Design review of the part built by this model. Coordinates are the model's own, in mm. A direction names the side the tool comes from. Coordinates: 2 decimals unless noted, no trailing zeros. Order: outer loops, then holes, each group sorted by start corner. A loop starts at its lowest first (then second) coordinate and runs counter-clockwise, first axis right, second up.
from build123d import *

# Parameters (mm, degrees)
F0_W     = 19.05
F0_H     = 120.65
F1_DEPTH = 127
F2_W     = 76.2
F2_H     = 76.2
F3_DEPTH = 76.2
F5_D     = 26.19502
F7_D     = 25.4


with BuildPart() as f1:
    # F0 (on Front) → F1 (new body)
    with BuildSketch(Plane.XZ):
        with BuildLine():
            ThreePointArc((120.65, 0), (85.3124331502, 85.3124331502), (0, 120.65))
            Line((0, 120.65), (0, 0))
            Line((0, 0), (120.65, 0))
        make_face()
        with Locations((-9.525, 60.325)):
            Rectangle(F0_W, F0_H)
    extrude(amount=-F1_DEPTH)

    # F2 (on face) → F3 (join)
    with BuildSketch(Plane(origin=(-19.05, 0, 0), x_dir=(0, -1, 0), z_dir=(-1, 0, 0))):
        with Locations((-38.1, 82.55)):
            Rectangle(F2_W, F2_H)
    extrude(amount=F3_DEPTH)

    # F5 (through all)
    with Locations(Plane(origin=(-95.25, 0, 0), x_dir=(0, -1, 0), z_dir=(-1, 0, 0))):
        with Locations((-38.1, 88.9)):
            Hole(F5_D / 2)

    # F7 (through all)
    with Locations(Plane.XZ):
        with Locations((57.15, 44.45)):
            Hole(F7_D / 2)


solid = f1.part
1. Add section D-D (y = 112). Give the boundary of the cut face in (x, z).
2. Add section B-B (x = 57.15). Give the boundary of the cut face in (y, z), and give its area (3 significant figures).
3. For faces 1 (the flat face through (-57, 76.2, 82)), 2 (the flat face through (50, 63, 0)), list the 3-axis set-ups (+Z, -Z, +X, -X, +Y, -Y) from which the entire face can be reached by the end or side of a thin tool; tool diameter is ignored.
4. Add section A-A (y = 38.1). Give the boundary of the cut face in (x, z).
5. Insertion check: pin 1 (4 mm diameter, centred on y = 90.5, z = 32.5, fed in from -X); pin 2 (1 mm diameter, centred on y = 18, z = 63, fed in from +X); pin 3 (5 mm diameter, centred on x = 8.5, z = 75.5, fed in from -Y); pin 4 (10 mm diameter, centred on x = -67.5, y = 25.5, fed in from -Z). Each pin has a flat end and moves straight along its axis. Give the tip position at first contact, or say it passes through.
6. Add section C-C (z = 51). Give the boundary of the cut face in (x, y).
7. To check wall thickness, follow line 1 (Z direction, x = -43.5, y = 38.1); line 2 (Y direction, x = 38, z = 88); line 3 (Z direction, x = 10.5, y = 38.1). State the ranges of each line that lie inside material, in increasing order.
8. Mouldability with a two-part tool opening along Y and no side actions: class faces 3 (the flat face through (-57, 39, 44.45)), 4 (the flat face through (34, 127, 61)), 5 (the cylindrical face through (0.63, 44.14, 77.28)) as pulls with the +Y half, pulls with the -Y half, needs draft (parallel to the pull), parting line crosses it, or undercut.
Solution:
1. outline: (-19.05, 0) - (120.65, 0) arc R120.65 ccw to (0, 120.65) - (-19.05, 120.65) - close; hole circle Ø25.4 at (57.15, 44.45)
2. outline: (0, 0) - (127, 0) - (127, 31.75) - (0, 31.75) - close; (0, 57.15) - (127, 57.15) - (127, 106.26) - (0, 106.26) - close; hole circle Ø26.2 at (38.1, 88.9)
2. area: 9,730 mm2
3. face 1: +Z, -Z, -X, +Y
3. face 2: -Z, +X, -X, +Y, -Y
4. outline: (-95.25, 44.45) - (-19.05, 44.45) - (-19.05, 0) - (120.65, 0) arc R120.65 ccw to (93.86, 75.8) - (-95.25, 75.8) - close; (-95.25, 102) - (64.44, 102) arc R120.65 ccw to (0, 120.65) - (-95.25, 120.65) - close; hole circle Ø25.4 at (57.15, 44.45)
5. pin 1: stops at x = -19.05
5. pin 2: stops at x = 103.2
5. pin 3: stops at y = 0
5. pin 4: stops at z = 44.45
6. outline: (-95.25, 0) - (46.27, 0) - (46.27, 127) - (-19.05, 127) - (-19.05, 76.2) - (-95.25, 76.2) - close; (68.03, 0) - (109.34, 0) - (109.34, 127) - (68.03, 127) - close
7. line 1: z = 44.45 to 75.8, 102 to 120.65
7. line 2: y = 0 to 25.03, 51.17 to 127
7. line 3: z = 0 to 75.8, 102 to 120.19
8. face 3: needs draft
8. face 4: pulls with the +Y half
8. face 5: undercut
